Part model, mm, in its own coordinate system. Face numbers are marked on the shaded views. Give positions to 0.01 mm unless a question says otherwise; leave off trailing zeros. Order: outer loops, then holes, each group sorted by start corner. A loop starts at its lowest first (then second) coordinate and runs counter-clockwise, first axis right, second up.
1. Probe line 1 (Z direction, x = -16, y = 31.5); line 2 (X direction, y = 46.5, z = 31); line 3 (X direction, y = 20.5, z = 130). List the from-to ranges inside material, lowest first.
2. Slice it at D-D on y = 39. List the corners of the cut face in (x, z).
3. Drop flat-ended pins along their axis: pin 1 Ø2.5 at (x, z) = (-75.5, 93) entering from -Y; pin 2 Ø5.5 at (y, z) = (-6, 92.5) entering from +X; pin 3 Ø1.5 at (y, z) = (18, 89.5) entering from +X. Give the stop position or say it passes through.
4. Slice it at B-B on y = 10.5. List the corners of the cut face in (x, z).
5. Slice it at A-A on z = 87.5. List the corners of the cut face in (x, y).
6. Mould opens along Z. For the marked faces 1, 2, 3 and 4 say: +Z half, -Z half, draft (parallel to the pull), parting line (faces both ways), or undercut.
7. Slice it at C-C on x = 39. List the corners of the cut face in (y, z), and give its area (3 significant figures).
from build123d import *

# Parameters (mm, degrees)
BOSS_EXTRUDE1_DEPTH = 160
SKETCH2_W           = 160
SKETCH2_H           = 140
CUT_EXTRUDE1_DEPTH  = 5
SHELL1_START        = 7.5
SHELL1_DEPTH        = 145


# Read off the part's stored shape, not the designer's step: Shell1
with BuildPart() as part:
    # Sketch1 → Boss-Extrude1 (new body)
    with BuildSketch(Plane.XY):
        Polygon((0, 61.386159038), (-80, 0), (-90, -7.67326988), (90, -7.67326988), (80, 0), align=None)
    extrude(amount=BOSS_EXTRUDE1_DEPTH)

    # Sketch2 → Cut-Extrude1 (cut)
    with BuildSketch(Plane.XZ.offset(7.67326988)):
        with Locations((0, 80)):
            Rectangle(SKETCH2_W, SKETCH2_H)
    extrude(amount=-CUT_EXTRUDE1_DEPTH, mode=Mode.SUBTRACT)

    # Shell1 outline → Shell1 (cut)
    with BuildSketch(Plane.XY.offset(SHELL1_START)):
        Polygon((0, 51.932615933), (-71.163775898, -2.67326988), (71.163775898, -2.67326988), align=None)
    extrude(amount=SHELL1_DEPTH, mode=Mode.SUBTRACT)


solid = part.part
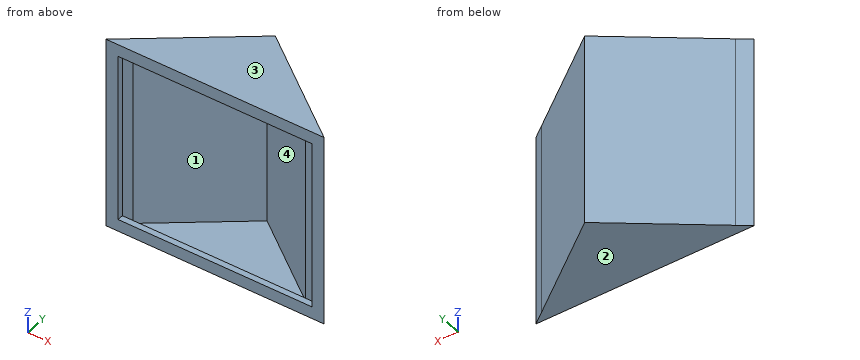
Data:
1. line 1: z = 0 to 7.5, 152.5 to 160
1. line 2: x = -19.4 to -7.08, 7.08 to 19.4
1. line 3: x = -53.28 to -40.96, 40.96 to 53.28
2. outline: (-29.17, 0) - (29.17, 0) - (29.17, 160) - (-29.17, 160) - close; hole (-16.85, 7.5) - (16.85, 7.5) - (16.85, 152.5) - (-16.85, 152.5) - close
3. pin 1: stops at y = -2.67
3. pin 2: stops at x = 90
3. pin 3: stops at x = 57.52
4. outline: (-66.32, 0) - (66.32, 0) - (66.32, 160) - (-66.32, 160) - close; hole (-54, 7.5) - (54, 7.5) - (54, 152.5) - (-54, 152.5) - close
5. outline: (-90, -7.67) - (-80, -7.67) - (-80, -2.67) - (-71.16, -2.67) - (0, 51.93) - (71.16, -2.67) - (80, -2.67) - (80, -7.67) - (90, -7.67) - (0, 61.39) - close
6. face 1: undercut
6. face 2: -Z half
6. face 3: +Z half
6. face 4: undercut
7. outline: (-7.67, 0) - (31.46, 0) - (31.46, 160) - (-7.67, 160) - (-7.67, 150) - (-2.67, 150) - (-2.67, 152.5) - (22.01, 152.5) - (22.01, 7.5) - (-2.67, 7.5) - (-2.67, 10) - (-7.67, 10) - close
7. area: 1,980 mm2
